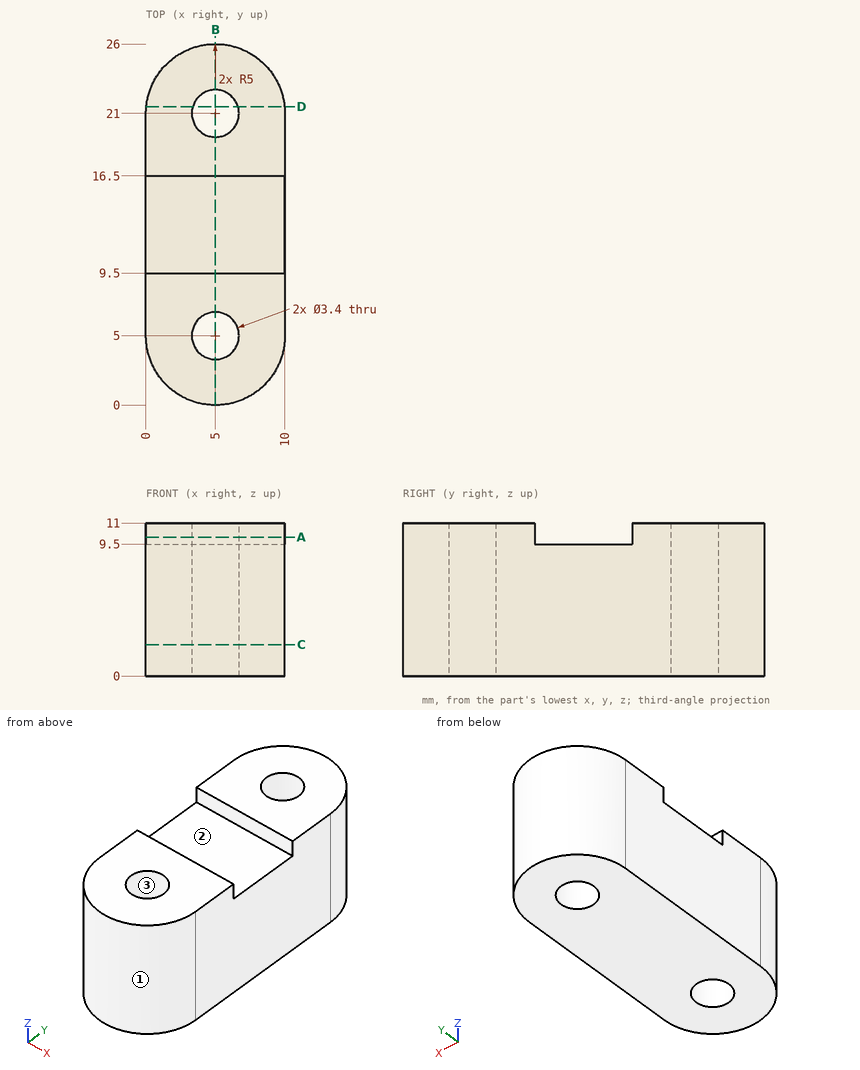
Can you work these out from the drawing? Everything is in mm from the part's minimum corner. Round coordinates to 2 decimals unless told otherwise and drop trailing zeros. Write each loop counter-clockwise with the first axis right and the second up, starting at its lowest first coordinate (ties: lowest second). Pieces come first, ordered by that corner, then holes. Notation, with made-up numbers: (-38, 82) - (14, 82) arc R19 ccw to (14, 88) - close; hole circle Ø7 at (-27.5, 75). An arc over 180 degrees is marked (long way). Use a Markdown table: item, result.
Q1. I want a section at B-B (x = 5). List the corners of the cut face in (y, z) for me, plus the area to 3 significant figures.
Output values:
| item | result |
|---|---|
| outline | (0, 0) - (3.3, 0) - (3.3, 11) - (0, 11) - close; (6.7, 0) - (19.3, 0) - (19.3, 11) - (16.5, 11) - (16.5, 9.5) - (9.5, 9.5) - (9.5, 11) - (6.7, 11) - close; (22.7, 0) - (26, 0) - (26, 11) - (22.7, 11) - close |
| area | 201 mm2 |
Q2. I want a section at C-C (z = 2.25). List the corners of the cut face in (x, y) for me, plus the area to 3 significant figures.
Output values:
| item | result |
|---|---|
| outline | (0, 5) arc R5 ccw to (10, 5) - (10, 21) arc R5 ccw to (0, 21) - close; hole circle Ø3.4 at (5, 5); hole circle Ø3.4 at (5, 21) |
| area | 220 mm2 |
Q3. Please list where these lines run through material, in increasing order: L1, parallel to Y at x = 5, z = 5; L2, parallel to Y at x = 4.5, z = 2; L3, parallel to Z at x = 9.75, y = 15.
Output values:
| item | result |
|---|---|
| L1 | 0 to 3.3, 6.7 to 19.3, 22.7 to 26 |
| L2 | 0.03 to 3.38, 6.62 to 19.38, 22.62 to 25.97 |
| L3 | 0 to 9.5 |
Q4. Thinking about a two-plate mould opening in X: for the marked faces 1, 2 and 3, which applies, released by +X, released by -X, zero draft, split by the parting line, or undercut?
Output values:
| item | result |
|---|---|
| face 1 | split by the parting line |
| face 2 | zero draft |
| face 3 | undercut |
Q5. For pin 1 (1 mm diameter, centred on x = 4, z = 1, fed in from -Y); pin 2 (0.8 mm diameter, centred on x = 3, z = 10, fed in from +Y); pin 3 (3 mm diameter, centred on x = 2, z = 4, fed in from +Y), each with a flat end and sliding along its axis, tell me the tip position at first contact or that it passes through.
Output values:
| item | result |
|---|---|
| pin 1 | y = 0.03 |
| pin 2 | y = 25.74 |
| pin 3 | y = 25.77 |
Q6. I want a section at A-A (z = 10). List the corners of the cut face in (x, y) for me, plus the area to 3 significant figures.
Output values:
| item | result |
|---|---|
| outline | (0, 5) arc R5 ccw to (10, 5) - (10, 9.5) - (0, 9.5) - close; (0, 16.5) - (10, 16.5) - (10, 21) arc R5 ccw to (0, 21) - close; hole circle Ø3.4 at (5, 5); hole circle Ø3.4 at (5, 21) |
| area | 150 mm2 |
Q7. I want a section at D-D (y = 21.5). List the corners of the cut face in (x, z) for me, plus the area to 3 significant figures.
Output values:
| item | result |
|---|---|
| outline | (0.03, 0) - (3.38, 0) - (3.38, 11) - (0.03, 11) - close; (6.62, 0) - (9.97, 0) - (9.97, 11) - (6.62, 11) - close |
| area | 73.7 mm2 |
